```python
from build123d import *

# Parameters (mm, degrees)
SKETCH006_W     = 105
SKETCH006_H     = 24
SKETCH006_R     = 4
PAD005_DEPTH    = 15
CHAMFER002_SIZE = 0.5
FILLET003_R     = 1


with BuildPart() as part:
    # Sketch006 → Pad005 (new body)
    with BuildSketch(Plane(origin=(100, 100, 0), x_dir=(1, 0, 0), z_dir=(0, 0, 1))):
        with Locations((0, 12)):
            Rectangle(SKETCH006_W, SKETCH006_H)
        with Locations((-35, 14)):
            Circle(SKETCH006_R, mode=Mode.SUBTRACT)
        with Locations((35, 14)):
            Circle(SKETCH006_R, mode=Mode.SUBTRACT)
    extrude(amount=PAD005_DEPTH)

    # Chamfer002
    chamfer002_edges = [part.edges().sort_by_distance(p)[0] for p in [
        (61, 114, 0),
        (131, 114, 0),
        (131, 114, 15),
        (61, 114, 15),
    ]]
    chamfer(chamfer002_edges, length=CHAMFER002_SIZE)

    # Fillet003
    fillet003_edges = [part.edges().sort_by_distance(p)[0] for p in [
        (152.5, 100, 7.5),
        (152.5, 124, 7.5),
        (152.5, 112, 0),
        (100, 100, 0),
        (100, 124, 0),
        (47.5, 100, 7.5),
        (47.5, 124, 7.5),
        (47.5, 112, 0),
    ]]
    fillet(fillet003_edges, radius=FILLET003_R)


solid = part.part
```
Verification items for the finished model (mm, model axes). Coordinates: 2 decimals unless noted, no trailing zeros. Loops run counter-clockwise (first coordinate to the right, second up) from the corner with the lowest first, then second, coordinate; pieces in that order, holes last. Notation, with made-up numbers: (85.5, -1.5) - (127.5, -1.5) arc R34 ccw to (127.5, 37.5) - close; hole circle Ø3 at (34, 49). An arc over 180 degrees is marked (long way). Put each result on its own line as item: value.
Item 1: Gauge pin test, flat end, axial feed: pin 1 Ø5 at (x, y) = (135, 114) entering from +Z. Record the tip position at first contact, or that the pin passes through.
Conclusion:
pin 1: passes through
Item 2: Section check A-A (x = 135). Enter the section's corners in (y, z), then the cut area to 3 significant figures.
Conclusion:
outline: (100, 1) arc R1 ccw to (101, 0) - (109.5, 0) - (110, 0.5) - (110, 14.5) - (109.5, 15) - (100, 15) - close; (118, 0.5) - (118.5, 0) - (123, 0) arc R1 ccw to (124, 1) - (124, 15) - (118.5, 15) - (118, 14.5) - close
area: 239 mm2
Item 3: Scan lines: line 1 along X through (y, z) = (112.5, 5.5); line 2 along X through (y, z) = (114.5, 3.75); line 3 along Y through (x, z) = (135, 6.75). Record each from-to range of solid material in increasing order.
Conclusion:
line 1: x = 47.5 to 61.29, 68.71 to 131.29, 138.71 to 152.5
line 2: x = 47.5 to 61.03, 68.97 to 131.03, 138.97 to 152.5
line 3: y = 100 to 110, 118 to 124
Item 4: Section check B-B (z = 7). Enter the section's corners in (x, y).
Conclusion:
outline: (47.5, 101) arc R1 ccw to (48.5, 100) - (151.5, 100) arc R1 ccw to (152.5, 101) - (152.5, 123) arc R1 ccw to (151.5, 124) - (48.5, 124) arc R1 ccw to (47.5, 123) - close; hole circle Ø8 at (65, 114); hole circle Ø8 at (135, 114)
Item 5: Section check C-C (y = 115). Give the number of separate pieces and of enclosed holes in the cut face, then the cut area to 3 significant figures.
Conclusion:
separate pieces: 3
enclosed holes: 0
area: 1,340 mm2
Item 6: Draft check along Y on faces 1 (the face through (99, 112, 0)), 2 (the face through (134.479, 117.966, 7.402)), 3 (the face through (99, 100, 8)), 4 (the face through (99, 124, 8)). Enter one of: pulls with the +Y half, pulls with the -Y half, needs draft (parallel to the pull), parting line crosses it, or undercut.
Conclusion:
face 1: needs draft
face 2: undercut
face 3: pulls with the -Y half
face 4: pulls with the +Y half
